Source: CAD feature listing. Evaluate the final solid. Frame: model axes, mm. Round coordinates to 2 decimals unless told otherwise and drop trailing zeros. Loops run counter-clockwise (first coordinate to the right, second up) from the corner with the lowest first, then second, coordinate; pieces in that order, holes last. Notation, with made-up numbers: M 39,-26 L 74,-26 A19 cw 74,1 Z; hole C 6,31 d11. An arc over 180 degrees is marked long. Answer as a JSON object with one key per item and string values.
from build123d import *

# Parameters (mm, degrees)
PAD_DEPTH                = 3
CHAMFER_SIZE             = 1
CHAMFER001_SIZE          = 1
BODY001_PLACEMENT_ANGLE  = 90
CLONE001_PLACEMENT_ANGLE = 90
BODY002_PLACEMENT_ANGLE  = 270
CLONE002_PLACEMENT_ANGLE = 270
BODY003_PLACEMENT_ANGLE  = 180


with BuildPart() as body:
    # Sketch → Pad (new body)
    with BuildSketch(Plane.XY):
        Polygon((-16.899492, 7.879108), (-16.899492, -7.879108), (16.899492, -7.879108), (16.899492, -20.39575), (34.896271, 0), (16.899492, 20.39575), (16.899492, 7.879108), align=None)
    extrude(amount=PAD_DEPTH)

    # Chamfer
    chamfer_edges = [body.edges().sort_by_distance(p)[0] for p in [
        (-16.899492, 0, 3),
        (0, -7.879108, 3),
        (16.899492, -14.137429, 3),
        (25.897881, -10.197875, 3),
        (25.897881, 10.197875, 3),
        (16.899492, 14.137429, 3),
        (0, 7.879108, 3),
    ]]
    chamfer(chamfer_edges, length=CHAMFER_SIZE)

    # Chamfer001
    chamfer001_edges = [body.edges().sort_by_distance(p)[0] for p in [
        (-16.899492, 0, 0),
        (0, -7.879108, 0),
        (16.899492, -14.137429, 0),
        (25.897881, -10.197875, 0),
        (25.897881, 10.197875, 0),
        (16.899492, 14.137429, 0),
        (0, 7.879108, 0),
    ]]
    chamfer(chamfer001_edges, length=CHAMFER001_SIZE)


with BuildPart() as body001:
    # Body001 base: copy of Body
    add(body.part)


with BuildPart() as body001_1:
    # Body001 placement: moved
    add(body001.part.moved(Location((-9, 9, 0))).rotate(Axis((-9, 9, 0), (0, 0, 1)), BODY001_PLACEMENT_ANGLE))


with BuildPart() as body002:
    # Body002 base: copy of Body001
    add(body001_1.part)


with BuildPart() as body002_1:
    # Clone001 placement: moved
    add(body002.part.moved(Location((-9, -9, 0))).rotate(Axis((-9, -9, 0), (0, 0, -1)), CLONE001_PLACEMENT_ANGLE))


with BuildPart() as body002_2:
    # Body002 placement: moved
    add(body002_1.part.moved(Location((-9, -9, 0))).rotate(Axis((-9, -9, 0), (0, 0, 1)), BODY002_PLACEMENT_ANGLE))


with BuildPart() as body003:
    # Body003 base: copy of Body002
    add(body002_2.part)


with BuildPart() as body003_1:
    # Clone002 placement: moved
    add(body003.part.moved(Location((-9, 9, 0))).rotate(Axis((-9, 9, 0), (0, 0, -1)), CLONE002_PLACEMENT_ANGLE))


with BuildPart() as body003_2:
    # Body003 placement: moved
    add(body003_1.part.moved(Location((-18, 0, 0))).rotate(Axis((-18, 0, 0), (0, 0, 1)), BODY003_PLACEMENT_ANGLE))


with BuildPart() as fusion:
    # Fusion base: copy of Body
    add(body.part)

    # Fusion: union Body001, Body002, Body003
    add(body001_1.part)
    add(body002_2.part)
    add(body003_2.part)


solid = fusion.part
Item 1: Contact query for flat-ended pins moving along their axis: pin 1 Ø1.1 at (y, z) = (12.5, 1.5) entering from +X; pin 2 Ø1.1 at (x, z) = (2, 1.5) entering from -Y; pin 3 Ø0.8 at (x, z) = (9, 1.5) entering from +Y; pin 4 Ø6 at (x, y) = (9.5, -20) entering from +Z. Output: stop coordinate, or through.
Answer sheet:
{"pin 1": "stops at x = 24.35", "pin 2": "stops at y = -34.68", "pin 3": "stops at y = 28.37", "pin 4": "passes through"}
Item 2: Section A-A on y = 19. Return the cut outline in (x, z).
Answer sheet:
{"outline": "M -36.13,1 L -35.43,0.47 L -34.9,1 L -34.9,2 L -35.43,2.53 L -36.13,2 Z; M -16.88,1 L -15.88,0 L -2.12,0 L -1.12,1 L -1.12,2 L -2.12,3 L -15.88,3 L -16.88,2 Z; M 16.9,1 L 17.43,0.47 L 18.13,1 L 18.13,2 L 17.43,2.53 L 16.9,2 Z"}
Item 3: Section D-D on x = -32. Return the cut outline in (y, z).
Answer sheet:
{"outline": "M -7.88,1 L -6.88,0 L 6.88,0 L 7.88,1 L 7.88,2 L 6.88,3 L -6.88,3 L -7.88,2 Z"}
Item 4: Line query: probe 1 along X at (y, z) = (-14.5, 2.15); probe 2 along Y at (x, z) = (3, 2.2); probe 3 along X at (y, z) = (19, 1.9). Output: solid intervals per line, ascending. Write a range as from..to.
Answer sheet:
{"probe 1": "x = -39.9..-35.05, -16.73..-1.27, 17.05..21.9", "probe 2": "y = -33.04..-26.1, -7.68..7.68, 26.1..33.04", "probe 3": "x = -36.13..-34.9, -16.88..-1.12, 16.9..18.13"}
Item 5: Section B-B on x = 1. Return the cut outline in (y, z).
Answer sheet:
{"outline": "M -35.07,1 L -33.74,0 L -26.9,0 L -25.9,1 L -25.9,2 L -26.9,3 L -33.74,3 L -35.07,2 Z; M -7.88,1 L -6.88,0 L 6.88,0 L 7.88,1 L 7.88,2 L 6.88,3 L -6.88,3 L -7.88,2 Z; M 25.9,1 L 26.9,0 L 33.74,0 L 35.07,1 L 35.07,2 L 33.74,3 L 26.9,3 L 25.9,2 Z"}
Item 6: Section C-C on z = 0.5. Return the cut outline in (x, y).
Answer sheet:
{"outline": "M -52.23,0 L -35.4,-19.07 L -35.4,-7.38 L -16.38,-7.38 L -16.38,-26.4 L -28.07,-26.4 L -9,-43.23 L 10.07,-26.4 L -1.62,-26.4 L -1.62,-7.38 L 17.4,-7.38 L 17.4,-19.07 L 34.23,0 L 17.4,19.07 L 17.4,7.38 L -1.62,7.38 L -1.62,26.4 L 10.07,26.4 L -9,43.23 L -28.07,26.4 L -16.38,26.4 L -16.38,7.38 L -35.4,7.38 L -35.4,19.07 Z"}
